from build123d import *

# Parameters (mm, degrees)
F1_DEPTH    = 5.08
F2_SIZE2    = 3.556
F2_SIZE     = 14.478
F3_T1_DEPTH = 183.3449978003
F4_R        = 10.16


# Not quite as in the source:
# - a fillet or chamfer that OpenCascade refuses, or shapes differently, is made with other operations: its cross-section is extruded or revolved along the edge and cut away or added


with BuildPart() as f1:
    # F0 (on Top) → F1 (new body)
    with BuildSketch(Plane.XY):
        Polygon((-38.1, 23.2852384394), (-19.05, -17.3547615606), (19.05, -17.3547615606), (38.1, 23.2852384394), align=None)
    extrude(amount=F1_DEPTH)

    # F2
    f2_edges = [f1.edges().sort_by_distance(p)[0] for p in [
        (0, 23.285238, 5.08),
    ]]
    f2_side = f1.faces().sort_by_distance((0, 5.223016, 5.08))[0]
    chamfer(f2_edges, length=F2_SIZE, length2=F2_SIZE2, reference=f2_side)

    # F3: chamfer of 27.94 x 3.556 on 1 edges, made by hand

    # F3_s2 → F3_t1 (cut)
    with BuildSketch(Plane.YZ.offset(-91.6724989001)):
        Polygon((10.5852384394, 5.08), (-17.3547615606, 1.524), (-17.3547615606, 5.08), align=None)
    extrude(amount=F3_T1_DEPTH, mode=Mode.SUBTRACT)

    # F4
    f4_edges = [f1.edges().sort_by_distance(p)[0] for p in [
        (19.05, -17.354762, 0.762),
        (-19.05, -17.354762, 0.762),
        (38.1, 23.285238, 0.762),
        (-38.1, 23.285238, 0.762),
    ]]
    fillet(f4_edges, radius=F4_R)


solid = f1.part
Source: CAD feature listing. Evaluate the final solid. Frame: model axes, mm. Give positions to 0.01 mm unless a question says otherwise; leave off trailing zeros. Write each loop counter-clockwise with the first axis right and the second up, starting at its lowest first coordinate (ties: lowest second). Pieces come first, ordered by that corner, then holes. Notation, with made-up numbers: (-18.5, 56) - (5.5, 56) arc R18 cw to (5.5, 74) - close; hole circle Ø8 at (59.5, 7). An arc over 180 degrees is marked (long way). Write item = value, one per line. Start each with the question number.
Q1. Cut plane A-A, the plane x = -9. Return loops of the section in (y, z).
Q2. Cut plane C-C, the plane y = 4. Return loops of the section in (x, z).
Q3. Pin query (flat end, axial travel): pin 1 Ø1.5 at (y, z) = (-1.5, 1) entering from -X. Return the tip coordinate at first contact, or that it passes through.
Q4. Draft query along X for faces 1 (the cylindrical face through (31.636, 16.676, 1.952)), 2 (the flat face through (-0.44, -3.78, 3.25)), 3 (the cylindrical face through (-18.11, -15.726, 0.898)). Return one class per face: +X half, -X half, draft (parallel to the pull), parting line (faces both ways), or undercut.
Q5. Cut plane D-D, the plane x = -19.5. Return loops of the section in (y, z).
Q6. Cut plane B-B, the plane z = 0.9. Return loops of the section in (x, y), then the cut area to 3 significant figures.
Q7. Material intervals for probe 1 along Y at (x, z) = (-19, 0.35); probe 2 along X at (y, z) = (-4, 3.1); probe 3 along X at (y, z) = (-2, 1.95), sorted ascending.
Computed values:
q1.outline = (-17.35, 0) - (23.29, 0) - (23.29, 1.52) - (9.41, 4.93) - (-17.35, 1.52) - close
q2.outline = (-29.06, 0) - (29.06, 0) - (29.06, 4.24) - (-29.06, 4.24) - close
q3.pin_1 = -26.83
q4.face_1 = +X half
q4.face_2 = draft
q4.face_3 = -X half
q5.outline = (-14.64, 0) - (23.29, 0) - (23.29, 1.52) - (9.41, 4.93) - (-14.64, 1.87) - close
q6.outline = (-31.32, 8.81) - (-21.79, -11.51) arc R10.16 ccw to (-12.59, -17.35) - (12.59, -17.35) arc R10.16 ccw to (21.79, -11.51) - (31.32, 8.81) arc R10.16 ccw to (22.12, 23.29) - (-22.12, 23.29) arc R10.16 ccw to start
q6.area = 2,190 mm²
q7.probe_1 = -15.08 to 23.29
q7.probe_2 = -25.31 to 25.31
q7.probe_3 = -26.25 to 26.25
